The model under review builds one solid part; all positions refer to its coordinate system, in mm. A direction names the side the tool comes from. Round coordinates to 2 decimals unless told otherwise and drop trailing zeros. Write each loop counter-clockwise with the first axis right and the second up, starting at its lowest first coordinate (ties: lowest second). Pieces come first, ordered by that corner, then holes. Notation, with made-up numbers: (60, -28.75) - (77, -28.75) arc R22 cw to (77, -14.75) - close; hole circle Ø10 at (44.5, -4.5). An arc over 180 degrees is marked (long way). Use one line per item in the form item = value.
from build123d import *

# Parameters (mm, degrees)
F1_DEPTH  = 10
F2_W      = 59.5
F2_H      = 56.5
F3_DEPTH  = 10.5
F5_DEPTH  = 59.501
F7_DEPTH  = 7
F8_R      = 3.1
F9_DEPTH  = 3.5
F10_R     = 3.1
F11_DEPTH = 3.5
F13_DEPTH = 10


with BuildPart() as f1:
    # F0 (on Top) → F1 (new body)
    with BuildSketch(Plane.XY):
        Polygon((23.75, -23.75), (23.75, 23.75), (-23.75, 23.75), (-23.75, -23.75), (-29.75, -29.75), (-29.75, -86.25), (29.75, -86.25), (29.75, -29.75), align=None)
    extrude(amount=F1_DEPTH)

    # F2 (on face) → F3 (join)
    with BuildSketch(Plane(origin=(0, 0, 0), x_dir=(1, 0, 0), z_dir=(0, 0, -1))):
        with Locations((0, 58)):
            Rectangle(F2_W, F2_H)
    extrude(amount=F3_DEPTH)

    # F4 (on face) → F5 (cut, through all)
    with BuildSketch(Plane.YZ.offset(29.75)):
        Polygon((-52.25, 0), (-42.25, 10), (-86.25, 10), (-86.25, 0), align=None)
        Polygon((-29.75, -10.5), (-29.75, 0), (-40.25, -10.5), align=None)
    extrude(amount=-F5_DEPTH, mode=Mode.SUBTRACT)

    # F6 (on face) → F7 (cut)
    with BuildSketch(Plane.XY):
        with BuildLine():
            ThreePointArc((-13.75, -66.25), (-19.25, -60.75), (-24.75, -66.25))
            Line((-24.75, -66.25), (-13.75, -66.25))
        make_face()
        with BuildLine():
            ThreePointArc((24.75, -66.25), (19.25, -60.75), (13.75, -66.25))
            Line((13.75, -66.25), (24.75, -66.25))
        make_face()
        with BuildLine():
            Line((24.75, -66.25), (13.75, -66.25))
            ThreePointArc((13.75, -66.25), (19.25, -71.75), (24.75, -66.25))
        make_face()
        with BuildLine():
            Line((-13.75, -66.25), (-24.75, -66.25))
            ThreePointArc((-24.75, -66.25), (-19.25, -71.75), (-13.75, -66.25))
        make_face()
    extrude(amount=-F7_DEPTH, mode=Mode.SUBTRACT)

    # F8 (on face) → F9 (cut, through all)
    with BuildSketch(Plane.XY.offset(-7)):
        with Locations((19.25, -66.25)):
            Circle(F8_R)
    extrude(amount=-F9_DEPTH, mode=Mode.SUBTRACT)

    # F10 (on face) → F11 (cut, through all)
    with BuildSketch(Plane.XY.offset(-7)):
        with Locations((-19.25, -66.25)):
            Circle(F10_R)
    extrude(amount=-F11_DEPTH, mode=Mode.SUBTRACT)

    # F12 (on face) → F13 (cut, through all)
    with BuildSketch(Plane.XY.offset(10)):
        with BuildLine():
            Line((-19.5, 18.4), (-19.5, 20))
            Line((-19.5, 20), (-17.9, 20))
            ThreePointArc((-17.9, 20), (-20.631371, 21.131371), (-19.5, 18.4))
        make_face()
        with BuildLine():
            Line((-17.9, 20), (-19.5, 20))
            Line((-19.5, 20), (-19.5, 18.4))
            ThreePointArc((-19.5, 18.4), (-18.368629, 18.868629), (-17.9, 20))
        make_face()
        with BuildLine():
            Line((19.5, 20), (17.9, 20))
            ThreePointArc((17.9, 20), (18.368629, 18.868629), (19.5, 18.4))
            Line((19.5, 18.4), (19.5, 20))
        make_face()
        with BuildLine():
            ThreePointArc((21.1, 20), (19.5, 21.6), (17.9, 20))
            Line((17.9, 20), (19.5, 20))
            Line((19.5, 20), (19.5, 18.4))
            ThreePointArc((19.5, 18.4), (20.631371, 18.868629), (21.1, 20))
        make_face()
        with BuildLine():
            ThreePointArc((-17.9, -20), (-18.368629, -18.868629), (-19.5, -18.4))
            Line((-19.5, -18.4), (-19.5, -20))
            Line((-19.5, -20), (-17.9, -20))
        make_face()
        with BuildLine():
            Line((-19.5, -20), (-19.5, -18.4))
            ThreePointArc((-19.5, -18.4), (-20.631371, -21.131371), (-17.9, -20))
            Line((-17.9, -20), (-19.5, -20))
        make_face()
        with BuildLine():
            Line((19.5, -20), (19.5, -18.4))
            ThreePointArc((19.5, -18.4), (18.368629, -18.868629), (17.9, -20))
            Line((17.9, -20), (19.5, -20))
        make_face()
        with BuildLine():
            ThreePointArc((21.1, -20), (20.631371, -18.868629), (19.5, -18.4))
            Line((19.5, -18.4), (19.5, -20))
            Line((19.5, -20), (17.9, -20))
            ThreePointArc((17.9, -20), (19.5, -21.6), (21.1, -20))
        make_face()
    extrude(amount=-F13_DEPTH, mode=Mode.SUBTRACT)


solid = f1.part
(1) Add section A-A on y = -66.25. Write out the cut boundary in (x, z), then the cut area to 3 significant figures.
Geometry results:
outline = (-29.75, -10.5) - (-22.35, -10.5) - (-22.35, -7) - (-24.75, -7) - (-24.75, 0) - (-29.75, 0) - close; (-16.15, -10.5) - (16.15, -10.5) - (16.15, -7) - (13.75, -7) - (13.75, 0) - (-13.75, 0) - (-13.75, -7) - (-16.15, -7) - close; (22.35, -10.5) - (29.75, -10.5) - (29.75, 0) - (24.75, 0) - (24.75, -7) - (22.35, -7) - close
area = 427 mm2
(2) The part is to be moulded in two halves that separate along Y. For faces 5 (the flat face through (0, -69, 0)), 6 (the cylindrical face through (-19.654, -63.176, -8.726)), 7 (the flat face through (0.42, -47.32, 4.93)), say which applies: +Y half, -Y half, draft (parallel to the pull), parting line (faces both ways), or undercut.
Geometry results:
face_5 = draft
face_6 = undercut
face_7 = -Y half
(3) Add section D-D on z = -8.5. Write out the cut boundary in (x, y).
Geometry results:
outline = (-29.75, -86.25) - (29.75, -86.25) - (29.75, -38.25) - (-29.75, -38.25) - close; hole circle Ø6.2 at (-19.25, -66.25); hole circle Ø6.2 at (19.25, -66.25)
(4) Insertion check: P1, Ø8, axis at y = -3.5, z = 7, coming from the -X side; P2, Ø6, axis at x = 18.5, z = -7.5, coming from the +Y side; P3, Ø10, axis at x = -1, z = -6.5, coming from the +Y side; P4, Ø10, axis at y = 8, z = -8, coming from the +X side. Each pin has a flat end and moves straight along its axis. Give the tip position at first contact, or say it passes through.
Geometry results:
P1 = -23.75
P2 = -34.25
P3 = -31.25
P4 = through
(5) Machinability: for faces 1 (the flat face through (0, -3, 0)), 2 (the flat face through (-17, -69, -7)), 3 (the flat face through (0, -86.25, -5)), 4 (the flat face through (23.75, 0, 5)), which of the approach directions +Z, -Z, +X, -X, +Y, -Y give a long, thin tool a straight path to every point of the face, cutting with its end or side? Answer none if there is none.
Geometry results:
face_1 = -Z, +X, -X, +Y
face_2 = +Z
face_3 = +Z, -Z, +X, -X, -Y
face_4 = +Z, -Z, +X, +Y
(6) Add section C-C on x = -8. Write out the cut boundary in (y, z), then the cut area to 3 significant figures.
Geometry results:
outline = (-86.25, -10.5) - (-40.25, -10.5) - (-29.75, 0) - (23.75, 0) - (23.75, 10) - (-42.25, 10) - (-52.25, 0) - (-86.25, 0) - close
area = 1,250 mm2
(7) To check wall thickness, follow L1, parallel to X at y = -20, z = 6; L2, parallel to Y at x = -19.5, z = 6.25; L3, parallel to Z at x = 2.5, y = -5. State the ranges of each line that lie inside material, in increasing order.
Geometry results:
L1 = -23.75 to -21.1, -17.9 to 17.9, 21.1 to 23.75
L2 = -46 to -21.6, -18.4 to 18.4, 21.6 to 23.75
L3 = 0 to 10
(8) Add section B-B on z = 8.75. Write out the cut boundary in (x, y).
Geometry results:
outline = (-29.75, -43.5) - (29.75, -43.5) - (29.75, -29.75) - (23.75, -23.75) - (23.75, 23.75) - (-23.75, 23.75) - (-23.75, -23.75) - (-29.75, -29.75) - close; hole circle Ø3.2 at (-19.5, -20); hole circle Ø3.2 at (-19.5, 20); hole circle Ø3.2 at (19.5, -20); hole (19.5, 18.4) arc R1.6 ccw to (21.1, 20) arc R1.6 ccw (long way) to start
